```python
from build123d import *

# Parameters (mm, degrees)
BOSS_EXTRUDE1_DEPTH = 26
BOSS_EXTRUDE2_DEPTH = 5


with BuildPart() as part:
    # Sketch1 → Boss-Extrude1 (new, symmetric)
    with BuildSketch(Plane.XY):
        with BuildLine():
            Line((42, 6.678571429), (42, 24.123084291))
            ThreePointArc((42, 24.123084291), (55.283419244, 32.092619283), (60.5, 46.678571429))
            Line((60.5, 46.678571429), (52.5, 46.678571429))
            ThreePointArc((52.5, 46.678571429), (37.5, 31.678571429), (22.5, 46.678571429))
            Line((22.5, 46.678571429), (14.5, 46.678571429))
            ThreePointArc((14.5, 46.678571429), (19.716580756, 32.092619283), (33, 24.123084291))
            Line((33, 24.123084291), (33, 6.678571429))
            Line((33, 6.678571429), (0, 6.678571429))
            Line((0, 6.678571429), (0, 0))
            Line((0, 0), (75, 0))
            Line((75, 0), (75, 6.678571429))
            Line((75, 6.678571429), (42, 6.678571429))
        make_face()
    extrude(amount=BOSS_EXTRUDE1_DEPTH, both=True)

    # Sketch1_3 → Boss-Extrude2 (add, symmetric)
    with BuildSketch(Plane.XY):
        with BuildLine():
            ThreePointArc((42, 24.123084291), (55.283419244, 32.092619283), (60.5, 46.678571429))
            Line((60.5, 46.678571429), (75, 6.678571429))
            Line((75, 6.678571429), (42, 6.678571429))
            Line((42, 6.678571429), (42, 24.123084291))
        make_face()
        with BuildLine():
            ThreePointArc((14.5, 46.678571429), (19.716580756, 32.092619283), (33, 24.123084291))
            Line((33, 24.123084291), (33, 6.678571429))
            Line((33, 6.678571429), (0, 6.678571429))
            Line((0, 6.678571429), (14.5, 46.678571429))
        make_face()
    extrude(amount=BOSS_EXTRUDE2_DEPTH, both=True)


solid = part.part
```
Geometry: final body of the model. Coordinates: model frame, mm. A direction names the side the tool comes from. Coordinates: 2 decimals unless noted, no trailing zeros. Write each loop counter-clockwise with the first axis right and the second up, starting at its lowest first coordinate (ties: lowest second). Pieces come first, ordered by that corner, then holes. Notation, with made-up numbers: M 50.25,34.25 L 64.25,34.25 A28 ccw 64.25,61.25 Z; hole C 33.5,72.25 d8. An arc over 180 degrees is marked long. Answer as CSV lines item,"result". Start each with the question number.
Q1. Reachability of faces 4 (the cylindrical face through (55.14, 31.92, 15.65)), 5 (the cylindrical face through (19.58, 32.26, 15.65)), 6 (the cylindrical face through (19.58, 32.26, -15.35)) from +Z, -Z, +X, -X, +Y, -Y: full face, straight path, thin tool, end or side. Return the list, or none.
Q2. Cut plane D-D on x = 66.5. Return the cut outline in (y, z).
Q3. Line query: line 1 (X direction, y = 13.5, z = -19); line 2 (Y direction, x = 7.5, z = -13); line 3 (X direction, y = 35.5, z = -2). Output: solid intervals per line, ascending. Write a range as from..to.
Q4. Mould query, pull axis Y, two halves, no side actions, for faces 1 (the flat face through (37, 18, -26)), 2 (the flat face through (33, 16, -15)), 3 (the flat face through (37, 0, 0)). Classes: released by +Y, released by -Y, zero draft, split by the parting line, or undercut.
Q5. Cut plane C-C on x = 59. Return the cut outline in (y, z), then the cut area to 3 significant figures.
Q6. Pin query (flat end, axial travel): P1, Ø5, axis at x = 16.5, y = 22, coming from the +Z side; P2, Ø16.5, axis at x = 65, y = 18, coming from the -Z side; P3, Ø14, axis at y = 14.5, z = 20.5, coming from the +X side. Return the tip coordinate at first contact, or that it passes through.
Q7. Cut plane A-A on y = 41. Return the cut outline in (x, z), then the cut area to 3 significant figures.
Q8. Cut plane B-B on z = -21. Return the cut outline in (x, y), then the cut area to 3 significant figures.
Findings below:
1,face 4,"+Z, +X"
1,face 5,"+Z, -X"
1,face 6,"-Z, -X"
2,outline,"M 0,-26 L 6.68,-26 L 6.68,-5 L 30.13,-5 L 30.13,5 L 6.68,5 L 6.68,26 L 0,26 Z"
3,line 1,"x = 33..42"
3,line 2,"y = 0..6.68"
3,line 3,"x = 10.45..27.5, 47.5..64.55"
4,face 1,"zero draft"
4,face 2,"undercut"
4,face 3,"released by -Y"
5,outline,"M 0,-26 L 6.68,-26 L 6.68,-5 L 38.51,-5 L 38.51,-26 L 46.68,-26 L 46.68,26 L 38.51,26 L 38.51,5 L 6.68,5 L 6.68,26 L 0,26 Z"
5,area,"1,090 mm2"
6,P1,"stops at z = 5"
6,P2,"stops at z = -5"
6,P3,"stops at x = 42"
7,outline,"M 12.44,-5 L 15.21,-5 L 15.21,-26 L 23.62,-26 L 23.62,26 L 15.21,26 L 15.21,5 L 12.44,5 Z; M 51.38,-26 L 59.79,-26 L 59.79,-5 L 62.56,-5 L 62.56,5 L 59.79,5 L 59.79,26 L 51.38,26 Z"
7,area,"929 mm2"
8,outline,"M 0,0 L 75,0 L 75,6.68 L 42,6.68 L 42,24.12 A23 ccw 60.5,46.68 L 52.5,46.68 A15 cw 22.5,46.68 L 14.5,46.68 A23 ccw 33,24.12 L 33,6.68 L 0,6.68 Z"
8,area,"1,130 mm2"
